Part model, mm, in its own coordinate system. A direction names the side the tool comes from. Coordinates: 2 decimals unless noted, no trailing zeros. Loops run counter-clockwise (first coordinate to the right, second up) from the corner with the lowest first, then second, coordinate; pieces in that order, holes last. Notation, with made-up numbers: M -37,62 L 1,62 A33 ccw 1,99 Z; hole C 41,10 d4. An arc over 180 degrees is marked long. Use a Markdown table: item, result. Add a question column.
1) Pull direction Z, two halves, no side cores. Call faces 4 (the cylindrical face through (-5.1, 3.31, 1.72)), 5 (the flat face through (0, 3, -3)), 6 (the cylindrical face through (-0.386, -6.044, -0.794)), 7 (the flat face through (-4.623, 0, 0)): released by +Z, released by -Z, zero draft, split by the parting line, or undercut.
2) Band-saw the part on C-C (z = 4.5). List the corners of the cut face in (x, y).
3) Pin check, flat tips, straight feed: pin 1 Ø1.5 at (x, z) = (23, -4.5) entering from +Y; pin 2 Ø4 at (x, z) = (10.5, 4) entering from +Y; pin 3 Ø5 at (x, y) = (14, -4.5) entering from +Z; pin 4 Ø3.5 at (y, z) = (-1, -1) entering from -X. Stop position of each tip, or through.
4) Band-saw the part on A-A (z = 0). List the corners of the cut face in (x, y) (3 decimals).
5) Wall check: probe 1 along Y at (x, z) = (-5.15, 0); probe 2 along X at (y, z) = (-1.5, -5.25); probe 3 along X at (y, z) = (-2.5, 3). Give the ranges that are in metal, low to high. Write a range as from..to.
6) Tool access for faces 1 (the cylindrical face through (21.93, 1.93, -2.52)), 2 (the flat face through (-0.762, 3, 4)), 3 (the flat face through (-3, -4.661, 0)): list every direction of +Z, -Z, +X, -X, +Y, -Y with a clear straight run to the whole face (end or side of a thin tool).
7) Band-saw the part on B-B (x = 28). List the corners of the cut face in (y, z) (3 decimals).
from build123d import *

# Parameters (mm, degrees)
EXTRUDE1_REACH = 54.353


with BuildPart() as part:
    # Sketch1 → base-Revolve (revolve)
    with BuildSketch(Plane.XY, mode=Mode.PRIVATE) as base_revolve_sk:
        Polygon((0, 6.096), (-0.762, 6.096), (-0.762, 4.6609), (-5.588, 4.6609), (-5.588, 3.72872), (-4.6228, 3.72872), (-4.6228, 0), (0, 0), (46.0502, 0), (46.0502, 3.175), (0, 3.175), align=None)
    revolve(base_revolve_sk.sketch.rotate(Axis((0, 0, 0), (1, 0, 0)), 90), axis=Axis((0, 0, 0), (1, 0, 0)))

    # Sketch15 → Extrude1 (add, up to next)
    with BuildSketch(Plane.ZY.offset(5.588), mode=Mode.PRIVATE) as extrude1_sk1:
        with BuildLine():
            ThreePointArc((-4.036457824, -2.330449967), (-4.6609, 3.6e-08), (-4.036457787, 2.33045003))
            Line((-4.036457787, 2.33045003), (-5.381943739, 0))
            Line((-5.381943739, 0), (-4.036457824, -2.330449967))
        make_face()
    extrude1_tool1 = extrude(extrude1_sk1.sketch, amount=-EXTRUDE1_REACH, mode=Mode.PRIVATE) - part.part
    # Sketch15 → Extrude1 (add, up to next)
    with BuildSketch(Plane.ZY.offset(5.588), mode=Mode.PRIVATE) as extrude1_sk2:
        with BuildLine():
            ThreePointArc((-4.036457787, 2.33045003), (-2.330449985, 4.036457813), (0, 4.6609))
            Line((0, 4.6609), (-2.69097187, 4.6609))
            Line((-2.69097187, 4.6609), (-4.036457787, 2.33045003))
        make_face()
    extrude1_tool2 = extrude(extrude1_sk2.sketch, amount=-EXTRUDE1_REACH, mode=Mode.PRIVATE) - part.part
    # Sketch15 → Extrude1 (add, up to next)
    with BuildSketch(Plane.ZY.offset(5.588), mode=Mode.PRIVATE) as extrude1_sk3:
        with BuildLine():
            ThreePointArc((0, 4.6609), (2.330450001, 4.036457804), (4.036457805, 2.330449998))
            Line((4.036457805, 2.330449998), (2.69097187, 4.6609))
            Line((2.69097187, 4.6609), (0, 4.6609))
        make_face()
    extrude1_tool3 = extrude(extrude1_sk3.sketch, amount=-EXTRUDE1_REACH, mode=Mode.PRIVATE) - part.part
    # Sketch15 → Extrude1 (add, up to next)
    with BuildSketch(Plane.ZY.offset(5.588), mode=Mode.PRIVATE) as extrude1_sk4:
        with BuildLine():
            Line((4.036457776, -2.330450049), (5.381943739, 0))
            Line((5.381943739, 0), (4.036457805, 2.330449998))
            ThreePointArc((4.036457805, 2.330449998), (4.502083684, 1.206329686), (4.6609, 0))
            ThreePointArc((4.6609, 0), (4.502083676, -1.206329715), (4.036457776, -2.330450049))
        make_face()
    extrude1_tool4 = extrude(extrude1_sk4.sketch, amount=-EXTRUDE1_REACH, mode=Mode.PRIVATE) - part.part
    # Sketch15 → Extrude1 (add, up to next)
    with BuildSketch(Plane.ZY.offset(5.588), mode=Mode.PRIVATE) as extrude1_sk5:
        with BuildLine():
            Line((2.69097187, -4.6609), (4.036457776, -2.330450049))
            ThreePointArc((4.036457776, -2.330450049), (2.330449975, -4.036457819), (0, -4.6609))
            Line((0, -4.6609), (2.69097187, -4.6609))
        make_face()
    extrude1_tool5 = extrude(extrude1_sk5.sketch, amount=-EXTRUDE1_REACH, mode=Mode.PRIVATE) - part.part
    # Sketch15 → Extrude1 (add, up to next)
    with BuildSketch(Plane.ZY.offset(5.588), mode=Mode.PRIVATE) as extrude1_sk6:
        with BuildLine():
            Line((-2.69097187, -4.6609), (0, -4.6609))
            ThreePointArc((0, -4.6609), (-2.330450017, -4.036457795), (-4.036457824, -2.330449967))
            Line((-4.036457824, -2.330449967), (-2.69097187, -4.6609))
        make_face()
    extrude1_tool6 = extrude(extrude1_sk6.sketch, amount=-EXTRUDE1_REACH, mode=Mode.PRIVATE) - part.part
    add(extrude1_tool1.solids().sort_by_distance((-5.588, 0, -4.817334))[0])
    add(extrude1_tool2.solids().sort_by_distance((-5.588, 4.171933, -2.408667))[0])
    add(extrude1_tool3.solids().sort_by_distance((-5.588, 4.171933, 2.408667))[0])
    add(extrude1_tool4.solids().sort_by_distance((-5.588, 0, 4.817334))[0])
    add(extrude1_tool5.solids().sort_by_distance((-5.588, -4.171933, 2.408667))[0])
    add(extrude1_tool6.solids().sort_by_distance((-5.588, -4.171933, -2.408667))[0])

    # Sketch8 → point_Cut-Revolve1 (revolve, cut)
    with BuildSketch(Plane.XY, mode=Mode.PRIVATE) as point_cut_revolve1_sk:
        Polygon((46.0502, 0), (46.5582, 0), (46.5582, 3.683), (44.488409787, 3.683), (44.488409787, 3.175), (46.0502, 2.2733), align=None)
    revolve(point_cut_revolve1_sk.sketch.rotate(Axis((0, 0, 0), (1, 0, 0)), 90), axis=Axis((0, 0, 0), (1, 0, 0)), mode=Mode.SUBTRACT)


solid = part.part
Entries:
| question | item | result |
|---|---|---|
| 1 | face 4 | undercut |
| 1 | face 5 | zero draft |
| 1 | face 6 | split by the parting line |
| 1 | face 7 | undercut |
| 2 | outline | M -5.59,-1.53 L -0.76,-1.53 L -0.76,-4.11 L 0,-4.11 L 0,4.11 L -0.76,4.11 L -0.76,1.53 L -5.59,1.53 Z |
| 3 | pin 1 | through |
| 3 | pin 2 | y = 2.47 |
| 3 | pin 3 | z = 2.47 |
| 3 | pin 4 | x = -4.62 |
| 4 | outline | M -5.588,-4.661 L -0.762,-4.661 L -0.762,-6.096 L 0,-6.096 L 0,-3.175 L 44.488,-3.175 L 46.05,-2.273 L 46.05,2.273 L 44.488,3.175 L 0,3.175 L 0,6.096 L -0.762,6.096 L -0.762,4.661 L -5.588,4.661 L -5.588,3.729 L -4.623,3.729 L -4.623,-3.729 L -5.588,-3.729 Z |
| 5 | probe 1 | -4.66..-3.73, 3.73..4.66 |
| 5 | probe 2 | -0.76..0 |
| 5 | probe 3 | -5.59..0 |
| 6 | face 1 | +X |
| 6 | face 2 | -X |
| 6 | face 3 | +Z, -Z, -X, -Y |
| 7 | outline | C 0,0 d6.35 |
